Design review of the part built by this model. Coordinates are the model's own, in mm. Give positions to 0.01 mm unless a question says otherwise; leave off trailing zeros. Loops run counter-clockwise (first coordinate to the right, second up) from the corner with the lowest first, then second, coordinate; pieces in that order, holes last.
from build123d import *

# Parameters (mm, degrees)
SKETCH3_R           = 24
SKETCH3_R_2         = 14.35
BOSS_EXTRUDE1_DEPTH = 15
CUT_EXTRUDE2_START  = 50
SKETCH4_R           = 1.5
CUT_EXTRUDE2_DEPTH  = 100
SKETCH5_R           = 1.5
CUT_EXTRUDE3_DEPTH  = 100
CUT_EXTRUDE6_DEPTH  = 26
CUT_EXTRUDE7_DEPTH  = 26
CUT_EXTRUDE8_DEPTH  = 26
CUT_EXTRUDE9_DEPTH  = 26
FILLET5_R           = 3


with BuildPart() as part:
    # Sketch3 → Boss-Extrude1 (new body)
    with BuildSketch(Plane(origin=(0, 0, 0), x_dir=(1, 0, 0), z_dir=(0, 1, 0))):
        Circle(SKETCH3_R)
        Circle(SKETCH3_R_2, mode=Mode.SUBTRACT)
    extrude(amount=BOSS_EXTRUDE1_DEPTH)

    # Sketch4 → Cut-Extrude2 (cut)
    with BuildSketch(Plane(origin=(0, 0, 0), x_dir=(0, 0, -1), z_dir=(1, 0, 0)).offset(CUT_EXTRUDE2_START)):
        with Locations((0, 7.5)):
            Circle(SKETCH4_R)
    extrude(amount=-CUT_EXTRUDE2_DEPTH, mode=Mode.SUBTRACT)

    # Sketch5 → Cut-Extrude3 (cut)
    with BuildSketch(Plane(origin=(0, 15, 0), x_dir=(1, 0, 0), z_dir=(0, 1, 0))):
        with Locations((0, 19.175)):
            Circle(SKETCH5_R)
        with Locations((0, -19.175)):
            Circle(SKETCH5_R)
    extrude(amount=-CUT_EXTRUDE3_DEPTH, mode=Mode.SUBTRACT)

    # Sketch7 → Cut-Extrude6 (cut)
    with BuildSketch(Plane(origin=(0, 15, 0), x_dir=(1, 0, 0), z_dir=(0, 1, 0))):
        with BuildLine():
            Line((3.5, 15.175), (3.5, 22.675))
            ThreePointArc((3.5, 22.675), (16.223526512, 16.223526512), (22.675, 3.5))
            Line((22.675, 3.5), (15.175, 3.5))
            ThreePointArc((15.175, 3.5), (11.012053056, 11.012053056), (3.5, 15.175))
        make_face()
    extrude(amount=-CUT_EXTRUDE6_DEPTH, mode=Mode.SUBTRACT)

    # Sketch9 → Cut-Extrude7 (cut)
    with BuildSketch(Plane(origin=(0, 15, 0), x_dir=(1, 0, 0), z_dir=(0, 1, 0))):
        with BuildLine():
            Line((15.175, -3.5), (22.675, -3.5))
            ThreePointArc((22.675, -3.5), (16.223526512, -16.223526512), (3.5, -22.675))
            Line((3.5, -22.675), (3.5, -15.175))
            ThreePointArc((3.5, -15.175), (11.012053056, -11.012053056), (15.175, -3.5))
        make_face()
    extrude(amount=-CUT_EXTRUDE7_DEPTH, mode=Mode.SUBTRACT)

    # Sketch10 → Cut-Extrude8 (cut)
    with BuildSketch(Plane(origin=(0, 15, 0), x_dir=(1, 0, 0), z_dir=(0, 1, 0))):
        with BuildLine():
            Line((-3.5, 15.175), (-3.5, 22.675))
            ThreePointArc((-3.5, 22.675), (-16.223526512, 16.223526512), (-22.675, 3.5))
            Line((-22.675, 3.5), (-15.175, 3.5))
            ThreePointArc((-15.175, 3.5), (-11.012053056, 11.012053056), (-3.5, 15.175))
        make_face()
    extrude(amount=-CUT_EXTRUDE8_DEPTH, mode=Mode.SUBTRACT)

    # Sketch11 → Cut-Extrude9 (cut)
    with BuildSketch(Plane(origin=(0, 15, 0), x_dir=(1, 0, 0), z_dir=(0, 1, 0))):
        with BuildLine():
            Line((-15.175, -3.5), (-22.675, -3.5))
            ThreePointArc((-22.675, -3.5), (-16.223526512, -16.223526512), (-3.5, -22.675))
            Line((-3.5, -22.675), (-3.5, -15.175))
            ThreePointArc((-3.5, -15.175), (-11.012053056, -11.012053056), (-15.175, -3.5))
        make_face()
    extrude(amount=-CUT_EXTRUDE9_DEPTH, mode=Mode.SUBTRACT)

    # Fillet5
    fillet5_edges = [part.edges().sort_by_distance(p)[0] for p in [
        (-3.5, 7.5, 22.675),
        (-22.675, 7.5, 3.5),
        (-15.175, 7.5, 3.5),
        (-3.5, 7.5, 15.175),
        (3.5, 7.5, -22.675),
        (22.675, 7.5, -3.5),
        (15.175, 7.5, -3.5),
        (3.5, 7.5, -15.175),
        (3.5, 7.5, 15.175),
        (15.175, 7.5, 3.5),
        (22.675, 7.5, 3.5),
        (3.5, 7.5, 22.675),
        (-3.5, 7.5, -15.175),
        (-15.175, 7.5, -3.5),
        (-22.675, 7.5, -3.5),
        (-3.5, 7.5, -22.675),
    ]]
    fillet(fillet5_edges, radius=FILLET5_R)


solid = part.part
Q1. Take a section at B-B (z = -2.5). Give the boundary of the cut face in (x, y), plus the area to 3 significant figures.
Results:
outline: (-23.87, 0) - (-14.13, 0) - (-14.13, 15) - (-23.87, 15) - close; (14.13, 0) - (23.87, 0) - (23.87, 15) - (14.13, 15) - close
area: 292 mm2
Q2. Draft analysis for pull direction X (two halves, no side actions). For faces 1 (the face through (22.89, 7.4, -7.21)), 2 (the face through (-21.32, 7.4, -4.79)), 3 (the face through (3.4, 0, 14.1)), state which applies: pulls with the +X half, pulls with the -X half, needs draft (parallel to the pull), parting line crosses it, or undercut.
Results:
face 1: parting line crosses it
face 2: undercut
face 3: needs draft
Q3. Wall thickness on line 1 (Z direction, x = 0, y = 6.75) (3 decimals); line 2 (X direction, y = 4, z = 5); line 3 (X direction, y = 7.5, z = 4.5): over which ranges is each line inside the solid? List them lowest first.
Results:
line 1: z = -24 to -20.675, -17.675 to -14.35, 14.35 to 17.675, 20.675 to 24
line 2: x = -23.47 to -21.45, -14.8 to -13.45, 13.45 to 14.8, 21.45 to 23.47
line 3: x = -23.57 to -21.09, -15.16 to -13.63, 13.63 to 15.16, 21.09 to 23.57
Q4. Take a section at A-A (x = 0). Give the boundary of the cut face in (y, z) (3 decimals).
Results:
outline: (0, -24) - (15, -24) - (15, -20.675) - (0, -20.675) - close; (0, -17.675) - (15, -17.675) - (15, -14.35) - (0, -14.35) - close; (0, 14.35) - (15, 14.35) - (15, 17.675) - (0, 17.675) - close; (0, 20.675) - (15, 20.675) - (15, 24) - (0, 24) - close
Q5. Take a section at C-C (x = -18). Give the boundary of the cut face in (y, z).
Results:
outline: (0, -15.87) - (15, -15.87) - (15, -14.23) - (0, -14.23) - close; (0, -3.5) - (15, -3.5) - (15, 3.5) - (0, 3.5) - close; (0, 14.23) - (15, 14.23) - (15, 15.87) - (0, 15.87) - close; hole circle Ø3 at (7.5, 0)
Q6. Insertion check: pin 1 (1.5 mm diameter, centred on x = -13.5, z = -11.5, fed in from +Y); pin 2 (1.6 mm diameter, centred on y = 10.5, z = 18.5, fed in from +X); pin 3 (1.2 mm diameter, centred on x = -18, y = 9.5, fed in from -Z); pin 4 (1.5 mm diameter, centred on y = 7.5, z = 10, fed in from +X). Each pin has a flat end and moves straight along its axis. Give the tip position at first contact, or say it passes through.
Results:
pin 1: passes through
pin 2: stops at x = 16.21
pin 3: stops at z = -16.53
pin 4: stops at x = 22.15
Q7. Take a section at D-D (y = 7.5). Give the number of separate pieces and of enclosed holes in the cut face, plus the area to 3 significant figures.
Results:
separate pieces: 2
enclosed holes: 6
area: 442 mm2
